Geometry check sheet. Reference: drawing and pictorial views, mm from the part's lowest x, y, z. A direction names the side the tool comes from. Round coordinates to 2 decimals unless told otherwise and drop trailing zeros. Write each loop counter-clockwise with the first axis right and the second up, starting at its lowest first coordinate (ties: lowest second). Pieces come first, ordered by that corner, then holes.
Item 1: Set-up check for the marked faces 4 and 5: record each of +Z, -Z, +X, -X, +Y, -Y from which the full face is reachable in a straight line by a thin tool's end or side.
Item 2: Section check C-C, the plane z = 29. Record the cut outline in (x, y), plus the area to 3 significant figures.
Item 3: Release check for a two-part mould opening along Y. For the marked faces 1, 2 and 3 record: pulls with the +Y half, pulls with the -Y half, needs draft (parallel to the pull), parting line crosses it, or undercut.
Item 4: Section check D-D, the plane y = 6. Record the cut outline in (x, z), plus the area to 3 significant figures.
Item 5: Material ranges on line 1 along X through (y, z) = (88.4, 19); line 2 along X through (y, z) = (70, 28); line 3 along Y through (x, z) = (22, 11), recorded low to high.
Item 6: Section check A-A, the plane x = 21. Record the cut outline in (y, z).
Item 7: Depth check by flat-ended pin: pin 1 (10.5 mm diameter, centred on x = 21, z = 19, fed in from -Y). Enter the tip coordinate at first touch or a pass-through.
Item 8: Section check B-B, the plane z = 19. Record the cut outline in (x, y), plus the area to 3 significant figures.
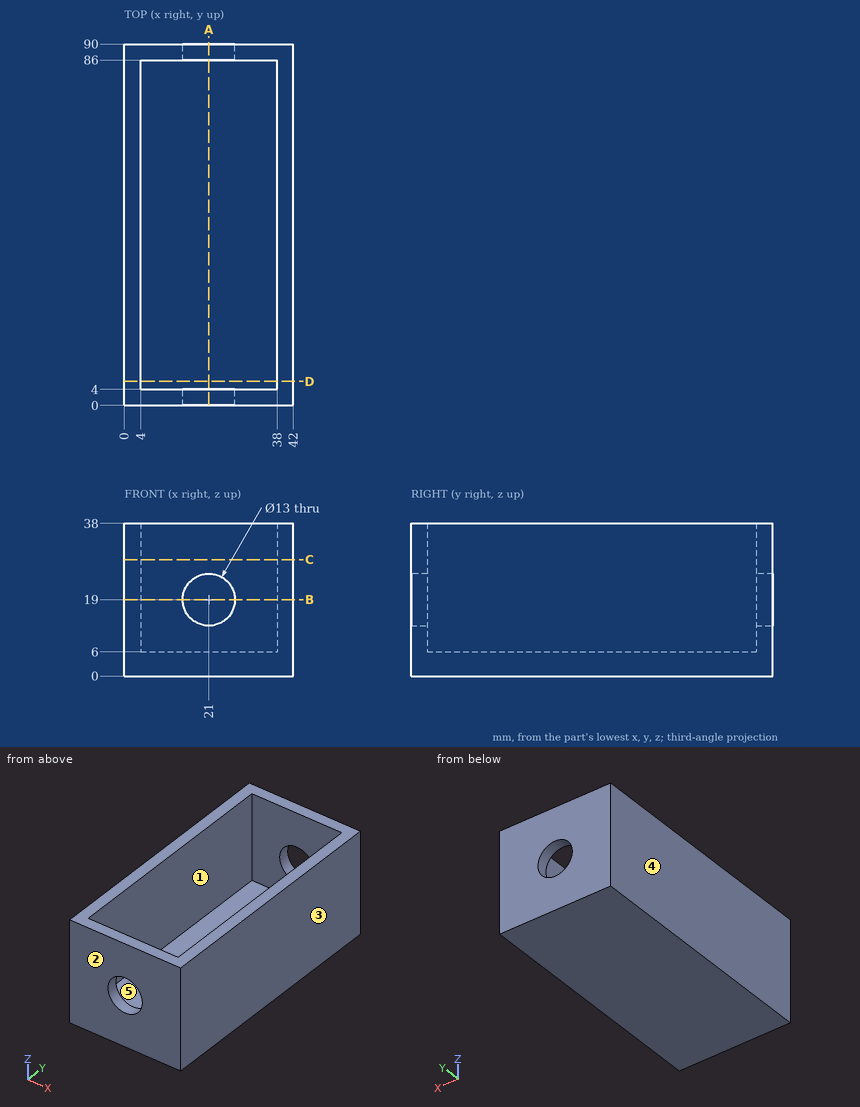
Values found:
1. face 4: +Z, -Z, -X, +Y, -Y
1. face 5: +Z
2. outline: (0, 0) - (42, 0) - (42, 90) - (0, 90) - close; hole (4, 4) - (38, 4) - (38, 86) - (4, 86) - close
2. area: 992 mm2
3. face 1: undercut
3. face 2: pulls with the -Y half
3. face 3: needs draft
4. outline: (0, 0) - (42, 0) - (42, 38) - (38, 38) - (38, 6) - (4, 6) - (4, 38) - (0, 38) - close
4. area: 508 mm2
5. line 1: x = 0 to 14.5, 27.5 to 42
5. line 2: x = 0 to 4, 38 to 42
5. line 3: y = 0 to 4, 86 to 90
6. outline: (0, 0) - (90, 0) - (90, 12.5) - (86, 12.5) - (86, 6) - (4, 6) - (4, 12.5) - (0, 12.5) - close; (0, 25.5) - (4, 25.5) - (4, 38) - (0, 38) - close; (86, 25.5) - (90, 25.5) - (90, 38) - (86, 38) - close
7. pin 1: passes through
8. outline: (0, 0) - (14.5, 0) - (14.5, 4) - (4, 4) - (4, 86) - (14.5, 86) - (14.5, 90) - (0, 90) - close; (27.5, 0) - (42, 0) - (42, 90) - (27.5, 90) - (27.5, 86) - (38, 86) - (38, 4) - (27.5, 4) - close
8. area: 888 mm2
